Source: CAD feature listing. Evaluate the final solid. Frame: model axes, mm. A direction names the side the tool comes from. Round coordinates to 2 decimals unless told otherwise and drop trailing zeros. Loops run counter-clockwise (first coordinate to the right, second up) from the corner with the lowest first, then second, coordinate; pieces in that order, holes last. Notation, with made-up numbers: (46, -35) -> (85, -35) arc R19 ccw to (85, -31) -> close; hole circle Ø3 at (30.5, 79). An arc over 180 degrees is marked (long way). Write item = value, one per line.
from build123d import *

# Parameters (mm, degrees)
SKETCH_1_W          = 25
SKETCH_1_H          = 25
EXTRUDE_1_DEPTH     = 4
SKETCH_2_W          = 19
SKETCH_2_H          = 19
CUT_EXTRUDE_1_DEPTH = 1
SKETCH_3_W          = 6
SKETCH_3_H          = 3.2
SKETCH_3_R          = 1.6
EXTRUDE_2_DEPTH     = 1
FILLET_1_R          = 1


with BuildPart() as part:
    # 草图1 → 凸台-拉伸1 (new body)
    with BuildSketch(Plane(origin=(0, 0, 0), x_dir=(1, 0, 0), z_dir=(0, 1, 0))):
        Rectangle(SKETCH_1_W, SKETCH_1_H)
    extrude(amount=EXTRUDE_1_DEPTH)

    # 草图2 → 切除-拉伸1 (cut)
    with BuildSketch(Plane(origin=(0, 4, 0), x_dir=(1, 0, 0), z_dir=(0, 1, 0))):
        Rectangle(SKETCH_2_W, SKETCH_2_H)
    extrude(amount=-CUT_EXTRUDE_1_DEPTH, mode=Mode.SUBTRACT)

    # 草图3 → 凸台-拉伸2 (add)
    # profile 1 of 3: a face of its own
    with BuildSketch(Plane(origin=(0, 3, 0), x_dir=(1, 0, 0), z_dir=(0, 1, 0))):
        Polygon((4.216148916, -1), (6, -1), (6, 1), (-6, 1), (-6, -1), (-4.216148916, -1), (-3.347471119, -6), (-4, -6), (-4, -8), (4, -8), (4, -6), (3.347471119, -6), align=None)
    # profile 2 of 3: a face of its own
    with BuildSketch(Plane(origin=(0, 3, 0), x_dir=(1, 0, 0), z_dir=(0, 1, 0))):
        with Locations((0, 3.1)):
            Rectangle(SKETCH_3_W, SKETCH_3_H)
        Polygon((-0.6, 3.933247604), (0, 4.4), (0.6, 3.933247604), (0, 2), align=None, mode=Mode.SUBTRACT)
    # profile 3 of 3: a face of its own
    with BuildSketch(Plane(origin=(0, 3, 0), x_dir=(1, 0, 0), z_dir=(0, 1, 0))):
        with Locations(Location((0, 6.394307769, 0), (0, 0, 270))):
            Circle(SKETCH_3_R)
    extrude(amount=EXTRUDE_2_DEPTH)

    # 圆角1
    fillet_1_edges = [part.edges().sort_by_distance(p)[0] for p in [
        (-9.5, 3.5, 9.5),
        (-9.5, 3.5, -9.5),
        (9.5, 3.5, -9.5),
        (9.5, 3.5, 9.5),
        (12.5, 2, 12.5),
        (-12.5, 2, 12.5),
        (-12.5, 2, -12.5),
        (12.5, 2, -12.5),
    ]]
    fillet(fillet_1_edges, radius=FILLET_1_R)


solid = part.part
1. Section query C-C (z = 4.75). Return the cut outline in (x, y).
Evaluation:
outline = (-12.5, 0) -> (12.5, 0) -> (12.5, 4) -> (9.5, 4) -> (9.5, 3) -> (3.56, 3) -> (3.56, 4) -> (-3.56, 4) -> (-3.56, 3) -> (-9.5, 3) -> (-9.5, 4) -> (-12.5, 4) -> close
2. Set-up query: faces 4 (the face through (-12.215, 2.028, 12.199)), 5 (the face through (-3.788, 3.493, 3.465)). Return all of +Z, -Z, +X, -X, +Y, -Y with unobstructed straight access to the full face (end or side cutting, diameter ignored); none if empty.
Evaluation:
face_4 = +Z, -X, +Y, -Y
face_5 = +Y
3. Section query B-B (y = 3.5). Give the number of separate pieces and of enclosed holes in the cut face, then the cut area to 3 significant figures.
Evaluation:
separate_pieces = 4
enclosed_holes = 2
area = 368 mm²
4. Section query A-A (x = -6.75). Return the cut outline in (y, z).
Evaluation:
outline = (0, -12.5) -> (4, -12.5) -> (4, -9.5) -> (3, -9.5) -> (3, 9.5) -> (4, 9.5) -> (4, 12.5) -> (0, 12.5) -> close
5. Line query: probe 1 along X at (y, z) = (3.45, -3.75); probe 2 along Z at (x, y) = (6.25, 3.1); probe 3 along X at (y, z) = (3.05, -7.25). Output: solid intervals per line, ascending. Write a range as from..to.
Evaluation:
probe_1 = -12.5..-9.5, -3..-0.54, 0.54..3, 9.5..12.5
probe_2 = -12.5..-9.5, 9.5..12.5
probe_3 = -12.5..-9.5, -1.35..1.35, 9.5..12.5
6. Mould query, pull axis X, two halves, no side actions, for faces 1 (the face through (12.199, 2.028, 12.215)), 2 (the face through (0, 0, 0)), 3 (the face through (0.304, 3.493, -2.98)). Classes: released by +X, released by -X, zero draft, split by the parting line, or undercut.
Evaluation:
face_1 = released by +X
face_2 = zero draft
face_3 = undercut
7. Section query D-D (x = 4.75). Return the cut outline in (y, z).
Evaluation:
outline = (0, -12.5) -> (4, -12.5) -> (4, -9.5) -> (3, -9.5) -> (3, -1) -> (4, -1) -> (4, 1) -> (3, 1) -> (3, 9.5) -> (4, 9.5) -> (4, 12.5) -> (0, 12.5) -> close
